Part model, mm, in its own coordinate system. Round coordinates to 2 decimals unless told otherwise and drop trailing zeros. Loops run counter-clockwise (first coordinate to the right, second up) from the corner with the lowest first, then second, coordinate; pieces in that order, holes last.
(1) Flat gauge pins, fed straight in: pin 1 (3 mm diameter, centred on x = -60, z = 0, fed in from +Y); pin 2 (1 mm diameter, centred on x = -28, y = 1.5, fed in from -Z). Where does each tip first touch, or does it go through?
(2) Cut at A-A on z = 18. List the corners of the cut face in (x, y), then the cut area to 3 significant figures.
(3) Cut at C-C on x = -60. List the corners of the cut face in (y, z), then the cut area to 3 significant figures.
(4) Cut at B-B on y = 3.25. List the corners of the cut face in (x, z).
(5) Cut at D-D on x = -17.5. List the corners of the cut face in (y, z), then the cut area to 3 significant figures.
(6) Probe probe 1 along X at (y, z) = (2.25, 1); probe 2 along Z at (x, y) = (51.5, 4); probe 3 along Z at (x, y) = (-60, 0.45). List the from-to ranges inside material, lowest first.
from build123d import *

# Parameters (mm, degrees)
SKETCH1_R           = 70
BOSS_EXTRUDE1_DEPTH = 8
CUT_EXTRUDE1_REACH  = 10
SKETCH2_R           = 2
SKETCH3_R           = 2.4
CUT_EXTRUDE2_DEPTH  = 2


with BuildPart() as part:
    # Sketch1 → Boss-Extrude1 (new body)
    with BuildSketch(Plane(origin=(0, 0, 0), x_dir=(1, 0, 0), z_dir=(0, 1, 0))):
        Circle(SKETCH1_R)
        with BuildLine():
            ThreePointArc((35, -29), (6, 0), (35, 29))
            ThreePointArc((35, 29), (55.506096654, 20.506096654), (64, 0))
            ThreePointArc((64, 0), (55.506096654, -20.506096654), (35, -29))
        make_face(mode=Mode.SUBTRACT)
    extrude(amount=BOSS_EXTRUDE1_DEPTH)

    # Sketch2 → Cut-Extrude1 (cut, up to next)
    with BuildSketch(Plane(origin=(0, 8, 0), x_dir=(1, 0, 0), z_dir=(0, 1, 0)), mode=Mode.PRIVATE) as cut_extrude1_sk1:
        with Locations((-59.999999981, -0.001490332)):
            Circle(SKETCH2_R)
    cut_extrude1_tool1 = extrude(cut_extrude1_sk1.sketch, amount=-CUT_EXTRUDE1_REACH, mode=Mode.PRIVATE) & part.part
    add(cut_extrude1_tool1.solids().sort_by_distance((-60, 8, 0.00149))[0], mode=Mode.SUBTRACT)

    # Sketch3 → Cut-Extrude2 (cut)
    with BuildSketch(Plane.XZ):
        with Locations((-59.999999981, 0.001490332)):
            Circle(SKETCH3_R)
    extrude(amount=-CUT_EXTRUDE2_DEPTH, mode=Mode.SUBTRACT)


solid = part.part
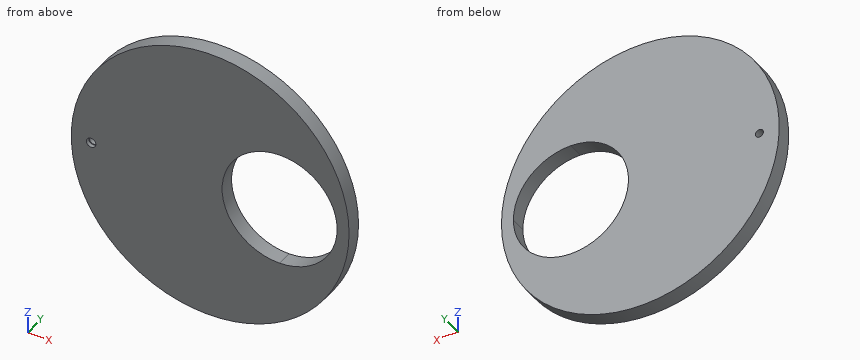
Final values:
1. pin 1: passes through
1. pin 2: stops at z = -64.37
2. outline: (-67.65, 0) - (12.26, 0) - (12.26, 8) - (-67.65, 8) - close; (57.74, 0) - (67.65, 0) - (67.65, 8) - (57.74, 8) - close
2. area: 719 mm2
3. outline: (0, -36.06) - (8, -36.06) - (8, -2) - (2, -2) - (2, -2.4) - (0, -2.4) - close; (0, 2.4) - (2, 2.4) - (2, 2) - (8, 2) - (8, 36.06) - (0, 36.06) - close
3. area: 543 mm2
4. outline: circle Ø140 at (0, 0); hole circle Ø4 at (-60, 0); hole circle Ø58 at (35, 0)
5. outline: (0, -67.78) - (8, -67.78) - (8, 67.78) - (0, 67.78) - close
5. area: 1,080 mm2
6. probe 1: x = -69.99 to -61.73, -58.27 to 6.02, 63.98 to 69.99
6. probe 2: z = -47.41 to -23.85, 23.85 to 47.41
6. probe 3: z = -36.06 to -2.4, 2.4 to 36.06
